Could you check a few things on this model? Use its own coordinates, in mm. A direction names the side the tool comes from. Round coordinates to 2 decimals unless told otherwise and drop trailing zeros. Write each loop counter-clockwise with the first axis right and the second up, starting at its lowest first coordinate (ties: lowest second). Pieces come first, ordered by that corner, then holes. Notation, with made-up numbers: M 60.5,76.5 L 107.5,76.5 A18 ccw 107.5,103.5 Z; hole C 41.5,20 d1. An arc over 180 degrees is marked long. One line per question, with ' | ' between items. Start each with the question number.
```python
from build123d import *

# Parameters (mm, degrees)
SKETCH1_W           = 250
SKETCH1_H           = 125
BOSS_EXTRUDE1_DEPTH = 35
SHELL1_T            = -10
SKETCH2_R           = 11
SKETCH2_R_2         = 7.5
SKETCH2_R_3         = 9
CUT_EXTRUDE1_DEPTH  = 70
FILLET1_R           = 1


with BuildPart() as part:
    # Sketch1 → Boss-Extrude1 (new body, symmetric)
    with BuildSketch(Plane.XY):
        with Locations((-130.188284519, 30.930962343)):
            Rectangle(SKETCH1_W, SKETCH1_H)
    extrude(amount=BOSS_EXTRUDE1_DEPTH, both=True)

    # Shell1
    shell1_openings = [part.faces().sort_by_distance(p)[0] for p in [
        (-5.188284519, 30.930962343, 0),
    ]]
    offset(amount=SHELL1_T, openings=shell1_openings, kind=Kind.INTERSECTION)

    # Sketch2 → Cut-Extrude1 (cut)
    with BuildSketch(Plane.XY.offset(35)):
        with Locations((-50, 30)):
            Circle(SKETCH2_R)
        with Locations((-104, 30)):
            Circle(SKETCH2_R_2)
        with Locations((-160.25, 30)):
            Circle(SKETCH2_R_3)
    extrude(amount=-CUT_EXTRUDE1_DEPTH, mode=Mode.SUBTRACT)

    # Fillet1
    fillet1_edges = [part.edges().sort_by_distance(p)[0] for p in [
        (-255.188284519, 30.930962343, 35),
        (-5.188284519, 30.930962343, -25),
        (-5.188284519, -21.569037657, 0),
        (-5.188284519, 83.430962343, 0),
        (-130.188284519, -31.569037657, 35),
        (-5.188284519, 30.930962343, 25),
        (-5.188284519, 30.930962343, 35),
        (-130.188284519, -31.569037657, -35),
        (-255.188284519, 30.930962343, -35),
        (-130.188284519, 93.430962343, -35),
        (-5.188284519, 30.930962343, -35),
        (-5.188284519, -31.569037657, 0),
        (-255.188284519, -31.569037657, 0),
        (-255.188284519, 93.430962343, 0),
        (-5.188284519, 93.430962343, 0),
        (-130.188284519, 93.430962343, 35),
    ]]
    fillet(fillet1_edges, radius=FILLET1_R)


solid = part.part
```
1. Suppose I cut it at D-D (z = -17). Write out the boundary of the cut face in (x, y).
2. Suppose I cut it at B-B (z = 30). Write out the boundary of the cut face in (x, y).
3. Suppose I cut it at C-C (y = 3). Write out the boundary of the cut face in (x, z), and give its area (3 significant figures).
4. Suppose I cut it at A-A (x = -104). Write out the boundary of the cut face in (y, z), and give its area (3 significant figures).
5. If we mould it in two halves opening along X, with no side actions, what happens to faces 3 (the face through (-5.188, 30, -30)), 4 (the face through (-39.839, 25.787, -29.93)), 5 (the face through (-127, 32, 25)), 6 (the face through (-255.188, 30, 0))? For each: released by +X, released by -X, zero draft, split by the parting line, or undercut.
6. Which directions (+Z, -Z, +X, -X, +Y, -Y) give clear straight access to the entire face, cutting with the end or side of a thin tool? Please do faces 1 (the face through (-169.24, 30.4, -29.93)), 2 (the face through (-127, 32, -25)).
7. I need wall thicknesses on line 1 along Z through (x, y) = (-231.5, 82.5); line 2 along Y through (x, z) = (-50, 31.5); line 3 along Y through (x, z) = (-160.25, -29.75). Which ranges of each line are inside material? Lowest first, please. Write a range as from..to.
Computed:
1) outline: M -255.19,-30.57 A1 ccw -254.19,-31.57 L -6.19,-31.57 A1 ccw -5.19,-30.57 L -5.19,-22.57 A1 ccw -6.19,-21.57 L -245.19,-21.57 L -245.19,83.43 L -6.19,83.43 A1 ccw -5.19,84.43 L -5.19,92.43 A1 ccw -6.19,93.43 L -254.19,93.43 A1 ccw -255.19,92.43 Z
2) outline: M -255.19,-30.57 A1 ccw -254.19,-31.57 L -6.19,-31.57 A1 ccw -5.19,-30.57 L -5.19,92.43 A1 ccw -6.19,93.43 L -254.19,93.43 A1 ccw -255.19,92.43 Z; hole C -160.25,30 d18; hole C -104,30 d15; hole C -50,30 d22
3) outline: M -255.19,-34 A1 ccw -254.19,-35 L -6.19,-35 A1 ccw -5.19,-34 L -5.19,-26 A1 ccw -6.19,-25 L -245.19,-25 L -245.19,25 L -6.19,25 A1 ccw -5.19,26 L -5.19,34 A1 ccw -6.19,35 L -254.19,35 A1 ccw -255.19,34 Z | area: 5,500 mm²
4) outline: M -31.57,-34 A1 ccw -30.57,-35 L 22.5,-35 L 22.5,-25 L -21.57,-25 L -21.57,25 L 22.5,25 L 22.5,35 L -30.57,35 A1 ccw -31.57,34 Z; M 37.5,-35 L 92.43,-35 A1 ccw 93.43,-34 L 93.43,34 A1 ccw 92.43,35 L 37.5,35 L 37.5,25 L 83.43,25 L 83.43,-25 L 37.5,-25 Z | area: 3,200 mm²
5) face 3: released by +X | face 4: undercut | face 5: zero draft | face 6: released by -X
6) face 1: +Z, -Z | face 2: +X
7) line 1: z = -35..-25, 25..35 | line 2: y = -31.57..19, 41..93.43 | line 3: y = -31.57..21, 39..93.43
